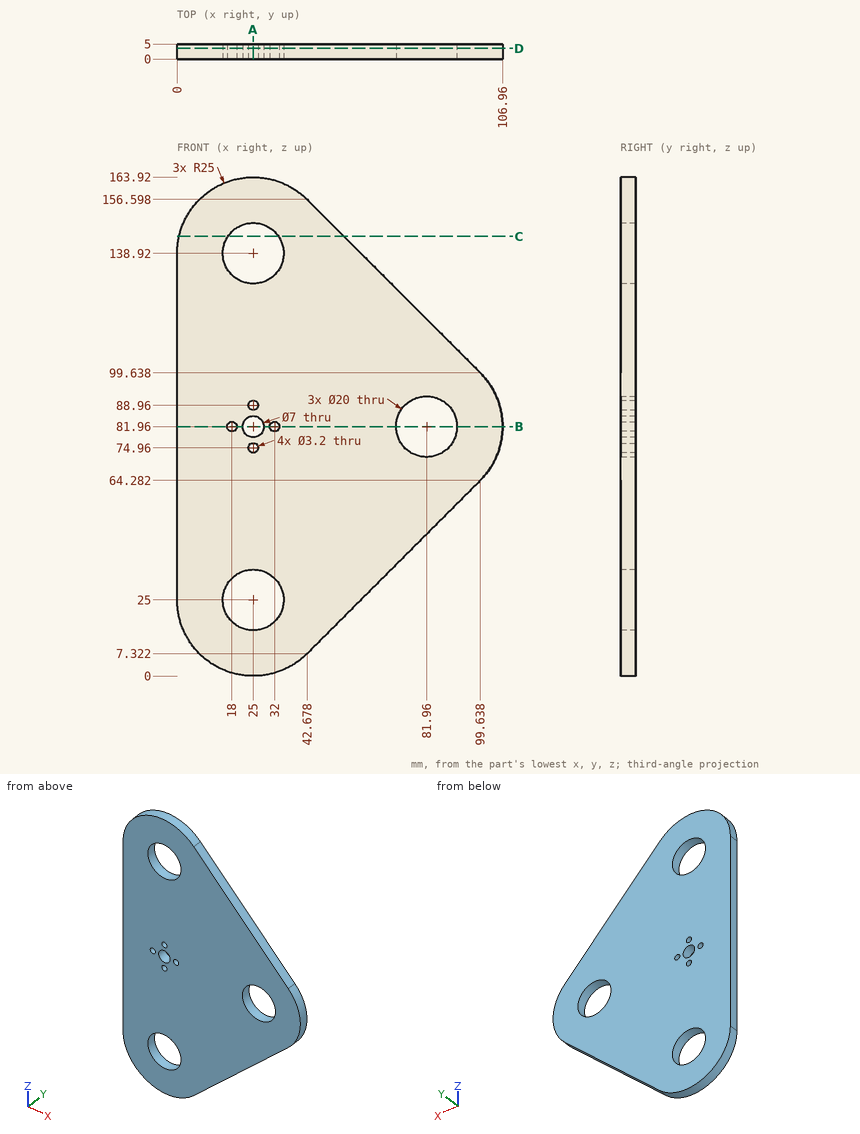
Answer from the drawing. Dimensions are ordinates in mm from the lowest x, y and z of the part. Coordinates: 2 decimals unless noted, no trailing zeros. Write each loop counter-clockwise with the first axis right and the second up, starting at its lowest first coordinate (ties: lowest second). Pieces come first, ordered by that corner, then holes. Notation, with made-up numbers: M 13.5,-7.75 L 66.5,-7.75 A30 ccw 66.5,27.25 Z; hole C 43.5,-15 d10. An arc over 180 degrees is marked long. Put each result on its own line as item: value. Start each with the question number.
1. A cutting plane is placed at D-D on y = 3.55. Count the separate pieces of the cut face and the enclosed holes in it, then the cut area to 3 significant figures.
2. A cutting plane is placed at C-C on z = 144.5. Write down the section's boundary in (x, y) (1 decimal), then the cut area to 3 significant figures.
3. A cutting plane is placed at B-B on z = 81.96. Write down the section's boundary in (x, y), then the cut area to 3 significant figures.
4. Flat-ended cylindrical pins translate along their axes: P1, Ø1, axis at x = 71, y = 1.5, coming from the -Z side (1 decimal); P2, Ø2, axis at x = 72, y = 1.5, coming from the -Z side (1 decimal); P3, Ø1.5, axis at y = 1, z = 24.5, coming from the -X side. Find the tip coordinate at first contact, or state that the pin passes through.
5. A cutting plane is placed at A-A on x = 25. Write down the section's boundary in (y, z).
6. Consider line 1 (X direction, y = 3.2, z = 81.96); line 2 (X direction, y = 2.2, z = 74.96); line 3 (Z direction, x = 90.5, y = 3.6) (1 decimal). Determine where each line is inside the solid, lowest interval first. Write a range as from..to.
Resolved:
1. separate pieces: 1
1. enclosed holes: 8
1. area: 11,100 mm2
2. outline: M 0.6,0 L 16.7,0 L 16.7,5 L 0.6,5 Z; M 33.3,0 L 54.8,0 L 54.8,5 L 33.3,5 Z
2. area: 188 mm2
3. outline: M 0,0 L 16.4,0 L 16.4,5 L 0,5 Z; M 19.6,0 L 21.5,0 L 21.5,5 L 19.6,5 Z; M 28.5,0 L 30.4,0 L 30.4,5 L 28.5,5 Z; M 33.6,0 L 71.96,0 L 71.96,5 L 33.6,5 Z; M 91.96,0 L 106.96,0 L 106.96,5 L 91.96,5 Z
3. area: 368 mm2
4. P1: stops at z = 35.1
4. P2: stops at z = 35.6
4. P3: stops at x = 0
5. outline: M 0,0 L 5,0 L 5,15 L 0,15 Z; M 0,35 L 5,35 L 5,73.36 L 0,73.36 Z; M 0,76.56 L 5,76.56 L 5,78.46 L 0,78.46 Z; M 0,85.46 L 5,85.46 L 5,87.36 L 0,87.36 Z; M 0,90.56 L 5,90.56 L 5,128.92 L 0,128.92 Z; M 0,148.92 L 5,148.92 L 5,163.92 L 0,163.92 Z
6. line 1: x = 0..16.4, 19.6..21.5, 28.5..30.4, 33.6..71.96, 91.96..106.96
6. line 2: x = 0..23.4, 26.6..74.82, 89.1..105.96
6. line 3: z = 55.1..76.8, 87.2..108.8
